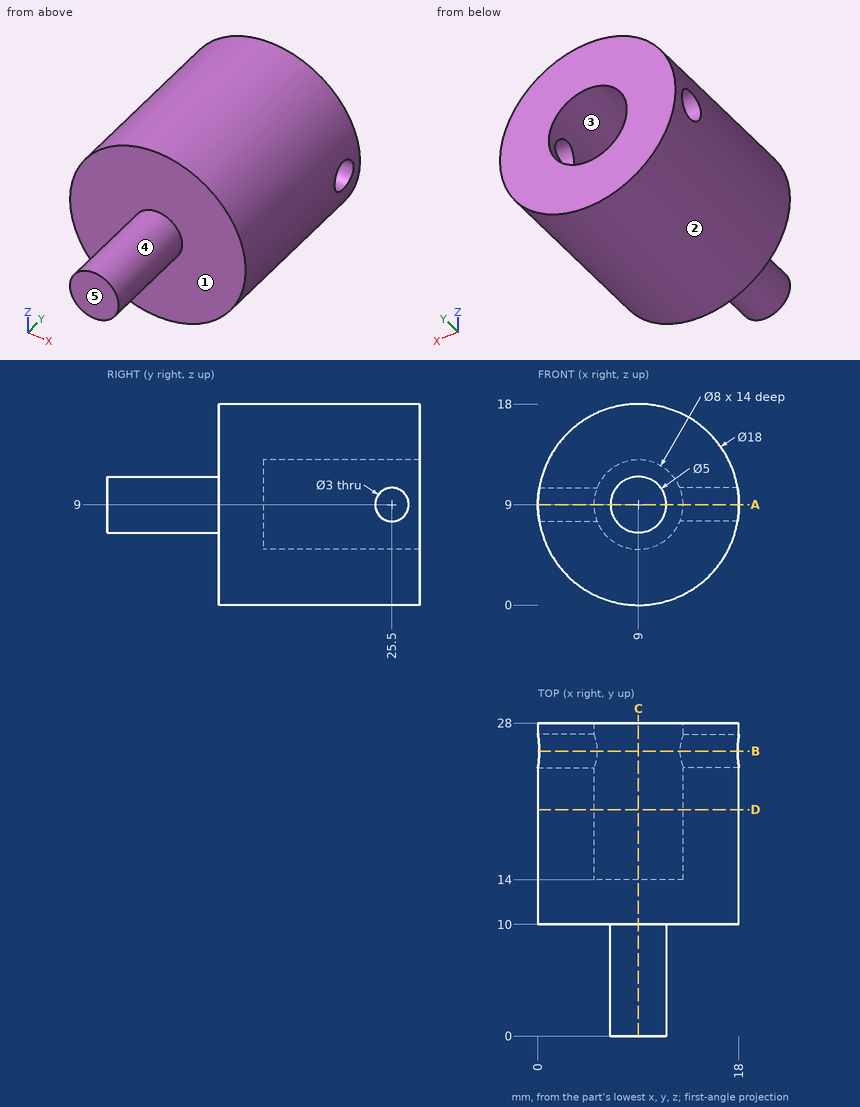
Print and shaded views of the part. All mm, measured from the part's lowest x, y and z. A direction names the side the tool comes from. Coordinates: 2 decimals unless noted, no trailing zeros. Write each loop counter-clockwise with the first axis right and the second up, starting at its lowest first coordinate (ties: lowest second). Pieces come first, ordered by that corner, then holes.
(1) Cut at B-B, the plane y = 25.5. List the corners of the cut face in (x, z).
(2) Cut at C-C, the plane x = 9. List the corners of the cut face in (y, z).
(3) Flat gauge pins, fed straight in: pin 1 (2 mm diameter, centred on x = 5.5, z = 11, fed in from -Y); pin 2 (6 mm diameter, centred on x = 2.5, y = 13, fed in from -Z); pin 3 (2 mm diameter, centred on x = 4, y = 12, fed in from +Z). Where does each tip first touch, or does it go through?
(4) Cut at D-D, the plane y = 20.25. List the corners of the cut face in (x, z), and give its area (3 significant figures).
(5) Two-plate mould, pull along Z, no slides. Class the marked faces 1, 2 and 3: +Z half, -Z half, draft (parallel to the pull), parting line (faces both ways), or undercut.
(6) 3-axis set-ups, long thin cutter, end or side, ignore diameter. For the marked faces 4 and 5: which of +Z, -Z, +X, -X, +Y, -Y reach the whole face in a straight line?
(7) Cut at A-A, the plane z = 9. List the corners of the cut face in (x, y), and give its area (3 significant figures).
(8) Drill centre lines: probe 1 along Z at (x, y) = (9, 17); probe 2 along Y at (x, z) = (7.75, 9.5); probe 3 along Y at (x, z) = (8.25, 1.25). Where is each one in solid material? Low to high.
Geometry says:
1. outline: (0.13, 7.5) arc R9 ccw to (17.87, 7.5) - (12.71, 7.5) arc R4 cw to (5.29, 7.5) - close; (0.13, 10.5) - (5.29, 10.5) arc R4 cw to (12.71, 10.5) - (17.87, 10.5) arc R9 ccw to start
2. outline: (0, 6.5) - (10, 6.5) - (10, 0) - (28, 0) - (28, 5) - (14, 5) - (14, 13) - (28, 13) - (28, 18) - (10, 18) - (10, 11.5) - (0, 11.5) - close
3. pin 1: stops at y = 10
3. pin 2: stops at z = 0.71
3. pin 3: stops at z = 17.06
4. outline: circle Ø18 at (9, 9); hole circle Ø8 at (9, 9)
4. area: 204 mm2
5. face 1: draft
5. face 2: parting line
5. face 3: undercut
6. face 4: -Y
6. face 5: +Z, -Z, +X, -X, -Y
7. outline: (0, 10) - (6.5, 10) - (6.5, 0) - (11.5, 0) - (11.5, 10) - (18, 10) - (18, 24) - (13, 24) - (13, 14) - (5, 14) - (5, 24) - (0, 24) - close; (0, 27) - (5, 27) - (5, 28) - (0, 28) - close; (13, 27) - (18, 27) - (18, 28) - (13, 28) - close
7. area: 232 mm2
8. probe 1: z = 0 to 5, 13 to 18
8. probe 2: y = 0 to 14
8. probe 3: y = 10 to 28
